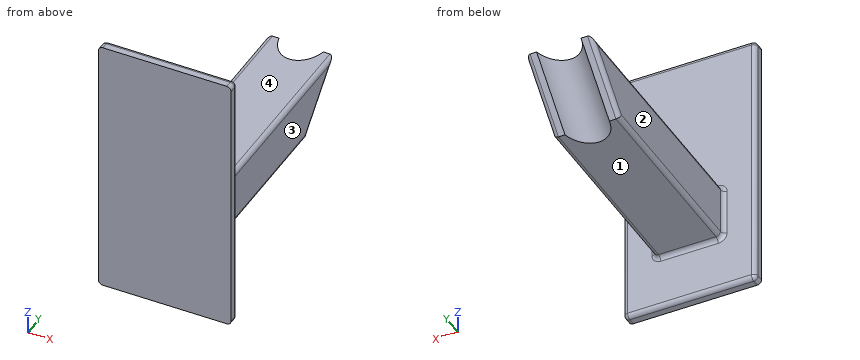
```python
from build123d import *

# Parameters (mm, degrees)
SKETCH1_W                = 76.2
SKETCH1_H                = 152.4
BOSS_EXTRUDE1_DEPTH      = 6.35
BOSS_EXTRUDE2_DEPTH      = 19.05
BOSS_EXTRUDE2_DEPTH_BACK = 19.05
SKETCH4_R                = 13.335
CUT_EXTRUDE1_DEPTH       = 175.596133978
FILLET1_R                = 2.54


with BuildPart() as part:
    # Sketch1 → Boss-Extrude1 (new body)
    with BuildSketch(Plane(origin=(0, 0, 0), x_dir=(1, 0, 0), z_dir=(0, 1, 0))):
        Rectangle(SKETCH1_W, SKETCH1_H)
    extrude(amount=BOSS_EXTRUDE1_DEPTH)

    # Sketch3 → Boss-Extrude2 (add, two sides: drawn at the far end of the back side and taken through both)
    with BuildSketch(Plane(origin=(0, 0, 0), x_dir=(0, 0, -1), z_dir=(1, 0, 0)).offset(-BOSS_EXTRUDE2_DEPTH_BACK)):
        Polygon((12.7, 6.35), (12.7, 152.4), (44.45, 120.65), (44.45, 6.35), align=None)
    extrude(amount=BOSS_EXTRUDE2_DEPTH + BOSS_EXTRUDE2_DEPTH_BACK)

    # Sketch4 → Cut-Extrude1 (cut, through all)
    with BuildSketch(Plane(origin=(0, 0, 0), x_dir=(1, 0, 0), z_dir=(0, 0.7071067811865486, 0.7071067811865465))):
        with Locations((0, 120.65)):
            Circle(SKETCH4_R)
    extrude(amount=CUT_EXTRUDE1_DEPTH, mode=Mode.SUBTRACT)

    # Fillet1
    fillet1_edges = [part.edges().sort_by_distance(p)[0] for p in [
        (-38.1, 6.35, 0),
        (0, 6.35, -44.45),
        (-19.05, 6.35, -28.575),
        (0, 6.35, -12.7),
        (19.05, 79.375, -12.7),
        (19.05, 136.525, -28.575),
        (0, 6.35, 76.2),
        (19.05, 63.5, -44.45),
        (-19.05, 79.375, -12.7),
        (-19.05, 136.525, -28.575),
        (-19.05, 63.5, -44.45),
        (19.05, 6.35, -28.575),
        (38.1, 6.35, 0),
        (38.1, 3.175, 76.2),
        (-38.1, 3.175, 76.2),
        (-38.1, 3.175, -76.2),
        (38.1, 3.175, -76.2),
        (0, 6.35, -76.2),
    ]]
    fillet(fillet1_edges, radius=FILLET1_R)


solid = part.part
```
Work out the finished part from the listing and answer in its coordinate system (mm). Face numbers are marked on the shaded views. A direction names the side the tool comes from. Round coordinates to 2 decimals unless told otherwise and drop trailing zeros. Write each loop counter-clockwise with the first axis right and the second up, starting at its lowest first coordinate (ties: lowest second). Pieces come first, ordered by that corner, then holes. Notation, with made-up numbers: (-35, -31) -> (18, -31) arc R23 ccw to (18, 8) -> close; hole circle Ø1 at (29.5, 46.25). An arc over 180 degrees is marked (long way). Write each question's results on one line, items separated by ' | '.
1) The part is cut by section A-A (y = 98). Write down the section's boundary in (x, z).
Findings:
outline: (-19.05, -41.91) arc R2.54 ccw to (-16.51, -44.45) -> (16.51, -44.45) arc R2.54 ccw to (19.05, -41.91) -> (19.05, -15.24) arc R2.54 ccw to (16.51, -12.7) -> (-16.51, -12.7) arc R2.54 ccw to (-19.05, -15.24) -> close
2) Consider line 1 along Y through (x, z) = (2.5, -56); line 2 along X through (y, z) = (133.5, -27); line 3 along Z through (x, y) = (3, 46). Determine where each line is inside the solid, lowest interval first. Write a range as [from, to].
Findings:
line 1: y = [0, 6.35] | line 2: x = [-19.05, -11.25], [11.25, 19.05] | line 3: z = [-44.45, -12.7]
3) The part is cut by section D-D (x = -25.5). Write down the section's boundary in (y, z), and give its area (3 significant figures).
Findings:
outline: (0, -76.2) -> (3.81, -76.2) arc R2.54 ccw to (6.35, -73.66) -> (6.35, 73.66) arc R2.54 ccw to (3.81, 76.2) -> (0, 76.2) -> close | area: 965 mm²
4) Flat-ended cylindrical pins translate along their axes: pin 1 (21.5 mm diameter, centred on y = 87.5, z = -27.5, fed in from +X); pin 2 (12 mm diameter, centred on x = -18, y = 42.5, fed in from -Z); pin 3 (21.5 mm diameter, centred on y = 94, z = -29.5, fed in from -X). Find the tip coordinate at first contact, or state that the pin passes through.
Findings:
pin 1: stops at x = 19.05 | pin 2: stops at z = -44.45 | pin 3: stops at x = -19.05
5) Which of the six approach directions +Z, -Z, +X, -X, +Y, -Y give full straight-line access (tool end or side, diameter ignored) to the marked faces 1, 2, 3 and 4?
Findings:
face 1: -Z, +X, -X, +Y | face 2: +Z, -Z, -X, +Y | face 3: +Z, -Z, +X, +Y | face 4: +Z, +X, -X, +Y
6) The part is cut by section C-C (z = -59). Write down the section's boundary in (x, y).
Findings:
outline: (-38.1, 0) -> (38.1, 0) -> (38.1, 3.81) arc R2.54 ccw to (35.56, 6.35) -> (-35.56, 6.35) arc R2.54 ccw to (-38.1, 3.81) -> close
7) The part is cut by section B-B (x = -0.5). Write down the section's boundary in (y, z).
Findings:
outline: (0, -76.2) -> (3.81, -76.2) arc R2.54 ccw to (6.35, -73.66) -> (6.35, -46.99) arc R2.54 cw to (8.89, -44.45) -> (107.33, -44.45) -> (139.08, -12.7) -> (8.89, -12.7) arc R2.54 cw to (6.35, -10.16) -> (6.35, 73.66) arc R2.54 ccw to (3.81, 76.2) -> (0, 76.2) -> close
